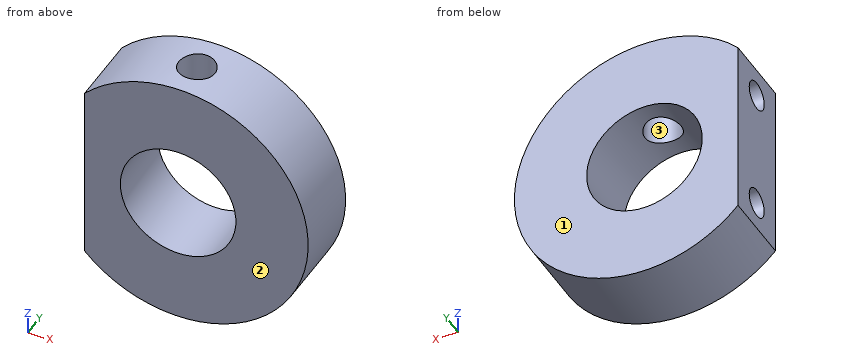
Autodesk Inventor part; units mm, degrees
ref_plane "XZ Plane" through (0, 0, 0) normal (0, 1, 0) x (-1, 0, 0)
ref_plane "XY Plane" through (0, 0, 0) normal (0, 0, 1) x (1, 0, 0)
sketch "Sketch1" plane through (0, 0, 0) normal (0, 1, 0) x (-1, 0, 0)
  circle A0 centre (0, 0) radius 8
  arc A1 (12.9518, 12.5) -> (12.9518, -12.5) centre (0, 0) ccw
  line L0 (12.9518, 12.5) -> (12.9518, -12.5)
  dimension "d0" = 16
  dimension "d13" = 36
  dimension "d14" = 25
extrude "Extrusion2" add sketch "Sketch1" along normal blind 10
sketch "Sketch3" plane through (-12.9518, 0, -12.5) normal (-1, 0, 0) x (0, 0, 1)
  circle A0 centre (21, 5) radius 2
  circle A1 centre (4, 5) radius 2
  line L0 (36, 5) -> (-7, 5) construction
  line L1 (25, 0) -> (0, 0)
  line L2 (25, 0) -> (25, 10)
  line L3 (0, 0) -> (0, 10)
  point P0 (12.5, 0)
  dimension "d17" = 4
  dimension "d18" = 4
  dimension "d19" = 5
  dimension "d20" = 17
  dimension "d21" = 4
  dimension "d22" = 25
extrude "Extrusion3" cut sketch "Sketch3" against normal blind 6
ref_plane "Work Plane2" through (0, 0, 0) normal (0, 0, -1) x (0, 1, 0)
sketch "Sketch4" plane through (0, 0, 0) normal (0, 0, -1) x (0, 1, 0)
  circle A0 centre (5, 0) radius 2.5
  point P0 (0, 0)
  dimension "d26" = 5
hole "Hole1" at (0, 5, 0) direction (0, 0, 1) diameter 5 end through all
equation "\"d21\" = -0.5 * d20 + 0.5 * d22"
properties part number "mocowanie uchwytu01"
Input: part model. Units: mm. Frame: model coordinates. Face numbers are marked on the shaded views. Coordinates: 2 decimals unless noted, no trailing zeros. Loops run counter-clockwise (first coordinate to the right, second up) from the corner with the lowest first, then second, coordinate; pieces in that order, holes last. Notation, with made-up numbers: M -25,-19.75 L -17,-19.75 A10 cw -17,-8.75 Z; hole C 76.5,71 d1. An arc over 180 degrees is marked long. Use a Markdown table: item, result. Add a question column.
1) Section A-A, the plane z = 0. Return the cut outline in (x, y).
2) Pin query (flat end, axial travel): P1, Ø1.5, axis at x = 11, y = 6, coming from the -Z side; P2, Ø1.5, axis at y = 9, z = 2.5, coming from the +X side; P3, Ø1.5, axis at x = 11.5, y = 6, coming from the -Z side. Return the tip coordinate at first contact, or that it passes through.
3) Draft query along Y for the marked faces 1, 2 and 3. Return one class per face: +Y half, -Y half, draft (parallel to the pull), parting line (faces both ways), or undercut.
4) Section B-B, the plane x = 0. Return the cut outline in (y, z).
5) Section C-C, the plane z = 13.5. Return the cut outline in (x, y).
6) Section D-D, the plane y = 1. Return the cut outline in (x, z), plus the area to 3 significant figures.
7) Line query: L1, parallel to Y at x = 0, z = 10; L2, parallel to Z at x = 0, y = 8; L3, parallel to Z at x = -11.5, y = 5.25. Output: solid intervals per line, ascending. Write a range as from..to.
Answer below:
| question | item | result |
|---|---|---|
| 1 | outline | M -12.95,0 L -8,0 L -8,10 L -12.95,10 Z; M 8,0 L 18,0 L 18,10 L 8,10 Z |
| 2 | P1 | z = -14.8 |
| 2 | P2 | x = 17.91 |
| 2 | P3 | z = -14.44 |
| 3 | face 1 | +Y half |
| 3 | face 2 | -Y half |
| 3 | face 3 | undercut |
| 4 | outline | M 0,-18 L 10,-18 L 10,-8 L 0,-8 Z; M 0,8 L 2.5,8 L 2.5,18 L 0,18 Z; M 7.5,8 L 10,8 L 10,18 L 7.5,18 Z |
| 5 | outline | M -11.91,0 L 11.91,0 L 11.91,10 L -11.91,10 Z; hole C 0,5 d5 |
| 6 | outline | M -12.95,-12.5 A18 ccw long -12.95,12.5 Z; hole C 0,0 d16 |
| 6 | area | 730 mm2 |
| 7 | L1 | 0..2.5, 7.5..10 |
| 7 | L2 | -18..-8, 8..18 |
| 7 | L3 | -13.85..-10.48, -6.52..6.52, 10.48..13.85 |
